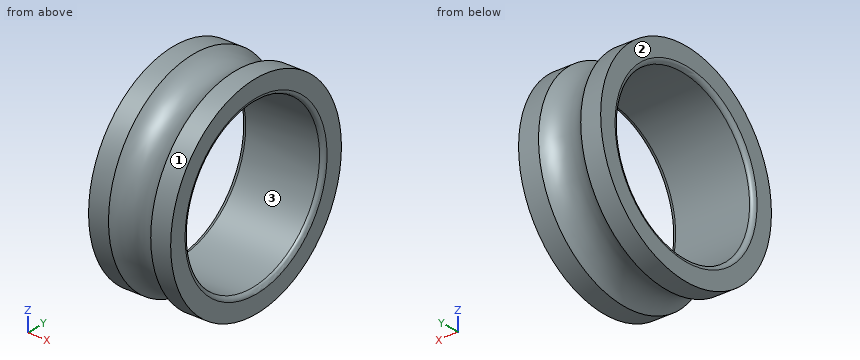
from build123d import *


with BuildPart() as part:
    # Esquisse1 → Base-Révolution (revolve)
    with BuildSketch(Plane.XY):
        with BuildLine():
            Line((0, 5.05), (0, 4.2))
            ThreePointArc((0, 4.2), (0.058578644, 4.058578644), (0.2, 4))
            Line((0.2, 4), (3.8, 4))
            ThreePointArc((3.8, 4), (3.941421356, 4.058578644), (4, 4.2))
            Line((4, 4.2), (4, 5.05))
            Line((4, 5.05), (3.02834819, 5.05))
            ThreePointArc((3.02834819, 5.05), (2, 4.6), (0.97165181, 5.05))
            Line((0.97165181, 5.05), (0, 5.05))
        make_face()
    revolve(axis=Axis((0, 0, 0), (1, 0, 0)))


solid = part.part
The listing builds one solid part. Answer for the finished solid, in the listing's coordinates (mm). Face numbers are marked on the shaded views. Give positions to 0.01 mm unless a question says otherwise; leave off trailing zeros. Order: outer loops, then holes, each group sorted by start corner. A loop starts at its lowest first (then second) coordinate and runs counter-clockwise, first axis right, second up. Notation, with made-up numbers: (-38, -12) -> (-26, -12) arc R16 cw to (-26, -7) -> close; hole circle Ø1 at (6.25, -22.5). An arc over 180 degrees is marked (long way). Put each result on its own line as item: value.
Item 1: Given P1, Ø2, axis at x = 1, y = 1.5, coming from the -Z side; P2, Ø5, axis at y = 0, z = 0, coming from the +X side; P3, Ø1.5, axis at y = -3.5, z = 0, coming from the -X side; P4, Ø1, axis at x = 1.5, z = -1, coming from the -Y side, each flat-ended and moving along its own axis, determine where each tip first touches the part or whether it passes through.
Established:
P1: stops at z = -5.03
P2: passes through
P3: stops at x = 0
P4: stops at y = -4.93
Item 2: A cutting plane is placed at D-D on x = 2.75. Give the vertices of the cut face in (y, z), plus the area to 3 significant figures.
Established:
outline: circle Ø9.64 at (0, 0); hole circle Ø8 at (0, 0)
area: 22.7 mm^2
Item 3: A cutting plane is placed at A-A on z = 0. Give the vertices of the cut face in (x, y).
Established:
outline: (0, -5.05) -> (0.97, -5.05) arc R1.4 cw to (3.03, -5.05) -> (4, -5.05) -> (4, -4.2) arc R0.2 ccw to (3.8, -4) -> (0.2, -4) arc R0.2 ccw to (0, -4.2) -> close; (0, 4.2) arc R0.2 ccw to (0.2, 4) -> (3.8, 4) arc R0.2 ccw to (4, 4.2) -> (4, 5.05) -> (3.03, 5.05) arc R1.4 cw to (0.97, 5.05) -> (0, 5.05) -> close
Item 4: Straight lines are drawn through the part: line 1 (Z direction, x = 2.8, y = 1.5); line 2 (Z direction, x = 1, y = 3.25); line 3 (Y direction, x = 2.1, z = 3.25). For each, find the intervals that lie inside material, in ascending order.
Established:
line 1: z = -4.61 to -3.71, 3.71 to 4.61
line 2: z = -3.83 to -2.33, 2.33 to 3.83
line 3: y = -3.26 to -2.33, 2.33 to 3.26
Item 5: A cutting plane is placed at C-C on x = 3.4. Give the vertices of the cut face in (y, z), plus the area to 3 significant figures.
Established:
outline: circle Ø10.1 at (0, 0); hole circle Ø8 at (0, 0)
area: 29.9 mm^2
Item 6: For a pull along Y with two mould halves and no side action, classify the marked faces 1, 2 and 3 as released by +Y, released by -Y, zero draft, split by the parting line, or undercut.
Established:
face 1: split by the parting line
face 2: zero draft
face 3: undercut
